Verification items for the finished model (mm, model axes). A direction names the side the tool comes from. Round coordinates to 2 decimals unless told otherwise and drop trailing zeros. Loops run counter-clockwise (first coordinate to the right, second up) from the corner with the lowest first, then second, coordinate; pieces in that order, holes last. Notation, with made-up numbers: (24, -21.75) - (63, -21.75) arc R13 cw to (63, -14.75) - close; hole circle Ø7 at (-18, -1). An arc over 180 degrees is marked (long way). Use CSV: the item, a comma, the result in double quotes.
```python
from build123d import *

# Parameters (mm, degrees)
BOSS_EXTRUDE5_DEPTH     = 67.31
CUT_EXTRUDE2_DEPTH      = 12.693340834
CUT_EXTRUDE3_DEPTH      = 25.4
SKETCH11_W              = 6.35
SKETCH11_H              = 25.4
BOSS_EXTRUDE6_DEPTH     = 6.35
SKETCH12_W              = 6.35
SKETCH12_H              = 25.4
CUT_EXTRUDE4_DEPTH      = 6.35
CUT_EXTRUDE5_DEPTH      = 171.430214526
CUT_EXTRUDE5_DEPTH_BACK = 6.35
SKETCH15_W              = 48.26
SKETCH15_H              = 27.94
CUT_EXTRUDE6_DEPTH      = 45.212


with BuildPart() as part:
    # Sketch1 → Boss-Extrude5 (new body)
    with BuildSketch(Plane(origin=(0, 0, 0), x_dir=(1, 0, 0), z_dir=(0, 1, 0))):
        Polygon((-60.605605599, 37.663504972), (95.096394401, 37.663504972), (95.096394401, 18.613504972), (-41.555605599, 18.613504972), (-41.555605599, -118.038495028), (-60.605605599, -118.038495028), align=None)
    extrude(amount=BOSS_EXTRUDE5_DEPTH)

    # Sketch8 → Cut-Extrude2 (cut)
    with BuildSketch(Plane(origin=(0, 67.31, 0), x_dir=(1, 0, 0), z_dir=(0, 1, 0))):
        Polygon((-57.303605599, -118.038495028), (-57.303605599, 34.361504972), (95.096394401, 34.361504972), (95.096394401, 31.059504972), (-54.001605599, 31.059504972), (-54.001605599, -118.038495028), align=None)
    extrude(amount=-CUT_EXTRUDE2_DEPTH, mode=Mode.SUBTRACT)

    # Sketch9 → Cut-Extrude3 (cut)
    with BuildSketch(Plane(origin=(0, 67.31, 0), x_dir=(1, 0, 0), z_dir=(0, 1, 0))):
        Polygon((-49.683605599, -118.038495028), (-49.683605599, 26.741504972), (95.096394401, 26.741504972), (95.096394401, 18.613504972), (-41.555605599, 18.613504972), (-41.555605599, -118.038495028), align=None)
    extrude(amount=-CUT_EXTRUDE3_DEPTH, mode=Mode.SUBTRACT)

    # Sketch11 → Boss-Extrude6 (add)
    with BuildSketch(Plane.XY.offset(118.038495028)):
        with Locations((-51.080605599, 12.7)):
            Rectangle(SKETCH11_W, SKETCH11_H)
    extrude(amount=BOSS_EXTRUDE6_DEPTH)

    # Sketch12 → Cut-Extrude4 (cut)
    with BuildSketch(Plane(origin=(95.096394401, 0, 0), x_dir=(0, 0, -1), z_dir=(1, 0, 0))):
        with Locations((28.138504972, 12.7)):
            Rectangle(SKETCH12_W, SKETCH12_H)
    extrude(amount=-CUT_EXTRUDE4_DEPTH, mode=Mode.SUBTRACT)

    # Sketch13 → Cut-Extrude5 (cut, two sides: drawn at the far end of the back side and taken through both)
    with BuildSketch(Plane.XZ.offset(-CUT_EXTRUDE5_DEPTH_BACK)):
        Polygon((-51.080605599, 570.867892173), (-51.080605599, 124.388495028), (-51.080605599, -25.399651713), (-51.080605599, -28.138504972), (88.746394401, -28.138504972), (535.225791546, -28.138504972), (1173.371683532, 596.477560176), (587.065286387, 1195.483957321), align=None)
    extrude(amount=CUT_EXTRUDE5_DEPTH + CUT_EXTRUDE5_DEPTH_BACK, mode=Mode.SUBTRACT)

    # Sketch15 → Cut-Extrude6 (cut)
    with BuildSketch(Plane(origin=(-41.555605599, 0, 0), x_dir=(0, 0, -1), z_dir=(1, 0, 0))):
        with Locations((-17.412502411, 25.379779706)):
            Rectangle(SKETCH15_W, SKETCH15_H)
    extrude(amount=-CUT_EXTRUDE6_DEPTH, mode=Mode.SUBTRACT)


solid = part.part
```
1) Mould release check, pull along Z, two halves, no side actions. Record for faces 4 (the face through (-52, 0, 7)), 5 (the face through (16, 33, -37.664)), 6 (the face through (-51, 25, 41.543)): +Z half, -Z half, draft (parallel to the pull), parting line (faces both ways), or undercut.
Returned:
face 4,"draft"
face 5,"-Z half"
face 6,"undercut"
2) Cross-section at D-D, the plane x = 43. Record the cut outline in (y, z).
Returned:
outline,"(0, -37.66) - (67.31, -37.66) - (67.31, -34.36) - (54.62, -34.36) - (54.62, -31.06) - (67.31, -31.06) - (67.31, -26.74) - (41.91, -26.74) - (41.91, -18.61) - (6.35, -18.61) - (6.35, -28.14) - (0, -28.14) - close"
3) Access from +Z, -Z, +X, -X, +Y, -Y to the whole of each face (thin tool, end or side, straight path). Record for faces 1 (the face through (-51, 25.4, 121)), 2 (the face through (-43, 6.35, 15)), 3 (the face through (18, 61, -34.362)).
Returned:
face 1,"+Z, +X, -X, +Y"
face 2,"+Z, +X, -Y"
face 3,"+X, +Y"
4) Gauge pin test, flat ends, axial feed: pin 1 Ø1.5 at (y, z) = (22.5, -6.5) entering from +X; pin 2 Ø1.9 at (y, z) = (9, 119.5) entering from -X; pin 3 Ø4 at (y, z) = (13.5, 22.5) entering from +X; pin 4 Ø20.5 at (x, y) = (46, 59) entering from +Z. Record the tip position at first contact, or that the pin passes through.
Returned:
pin 1,"stops at x = -41.56"
pin 2,"stops at x = -54.26"
pin 3,"passes through"
pin 4,"stops at z = -26.74"
5) Thickness scan on probe 1 along X at (y, z) = (64.5, -3.5); probe 2 along Z at (x, y) = (1, 63); probe 3 along Z at (x, y) = (77, 34). Record the ranges inside material, lowest first. Write a range as [from, to].
Returned:
probe 1,"x = [-60.61, -57.3], [-54, -49.68]"
probe 2,"z = [-37.66, -34.36], [-31.06, -26.74]"
probe 3,"z = [-37.66, -18.61]"
6) Cross-section at C-C, the plane x = -45.5. Record the cut outline in (y, z), then the cut area to 3 significant figures.
Returned:
outline,"(0, -37.66) - (67.31, -37.66) - (67.31, -34.36) - (54.62, -34.36) - (54.62, -31.06) - (67.31, -31.06) - (67.31, -26.74) - (41.91, -26.74) - (41.91, 118.04) - (6.35, 118.04) - (6.35, -28.14) - (0, -28.14) - close; hole (11.41, -6.72) - (39.35, -6.72) - (39.35, 41.54) - (11.41, 41.54) - close"
area,"4,480 mm²"
7) Cross-section at A-A, the plane y = 27.5. Record the cut outline in (x, z).
Returned:
outline,"(-60.61, -37.66) - (95.1, -37.66) - (95.1, -18.61) - (-41.56, -18.61) - (-41.56, -6.72) - (-60.61, -6.72) - close; (-60.61, 41.54) - (-41.56, 41.54) - (-41.56, 118.04) - (-60.61, 118.04) - close"
8) Cross-section at B-B, the plane z = 2.5. Record the cut outline in (x, y), then the cut area to 3 significant figures.
Returned:
outline,"(-60.61, 0) - (-51.08, 0) - (-51.08, 6.35) - (-41.56, 6.35) - (-41.56, 11.41) - (-60.61, 11.41) - close; (-60.61, 39.35) - (-41.56, 39.35) - (-41.56, 41.91) - (-49.68, 41.91) - (-49.68, 67.31) - (-54, 67.31) - (-54, 54.62) - (-57.3, 54.62) - (-57.3, 67.31) - (-60.61, 67.31) - close"
area,"441 mm²"
